```python
from build123d import *

# Parameters (mm, degrees)
SKETCH_1_R      = 2.25
SKETCH_1_R_2    = 2.075
EXTRUDE_1_DEPTH = 2.4
SKETCH_4_R      = 3.5
SKETCH_4_R_2    = 2.075
EXTRUDE_2_DEPTH = 9.9
FILLET_1_R      = 1
SKETCH_5_R      = 2.075
SKETCH_5_R_2    = 1.2
EXTRUDE_3_DEPTH = 4


with BuildPart() as part:
    # 草图1 → 凸台-拉伸1 (new body)
    with BuildSketch(Plane(origin=(0, 0, 0), x_dir=(0, 0, -1), z_dir=(1, 0, 0))):
        with BuildLine():
            Line((-5, 0), (5, 0))
            ThreePointArc((5, 0), (10, 5), (5, 10))
            Line((5, 10), (5, 21.282156306))
            ThreePointArc((5, 21.282156306), (0, 26.282156306), (-5, 21.282156306))
            Line((-5, 21.282156306), (-5, 10))
            ThreePointArc((-5, 10), (-10, 5), (-5, 0))
        make_face()
        with Locations((-5, 5)):
            Circle(SKETCH_1_R, mode=Mode.SUBTRACT)
        with Locations((5, 5)):
            Circle(SKETCH_1_R, mode=Mode.SUBTRACT)
        with Locations((0, 21.282156306)):
            Circle(SKETCH_1_R_2, mode=Mode.SUBTRACT)
    extrude(amount=EXTRUDE_1_DEPTH)

    # 草图4 → 凸台-拉伸2 (add)
    with BuildSketch(Plane(origin=(2.4, 0, 0), x_dir=(0, 0, -1), z_dir=(1, 0, 0))):
        with Locations(Location((0, 21.282156306, 0), (0, 0, 180))):
            Circle(SKETCH_4_R)
        with Locations((0, 21.282156306)):
            Circle(SKETCH_4_R_2, mode=Mode.SUBTRACT)
    extrude(amount=EXTRUDE_2_DEPTH)

    # 圆角1
    fillet_1_edges = [part.edges().sort_by_distance(p)[0] for p in [
        (2.4, 21.282156306, -3.5),
    ]]
    fillet(fillet_1_edges, radius=FILLET_1_R)

    # 草图5 → 凸台-拉伸3 (add)
    with BuildSketch(Plane.ZY):
        with Locations((0, 21.282156306)):
            Circle(SKETCH_5_R)
        with Locations((0, 21.282156306)):
            Circle(SKETCH_5_R_2, mode=Mode.SUBTRACT)
    extrude(amount=-EXTRUDE_3_DEPTH)


solid = part.part
```
For this review, take the finished solid that the model builds, in its own axes (mm). A direction names the side the tool comes from. Coordinates: 2 decimals unless noted, no trailing zeros. Write each loop counter-clockwise with the first axis right and the second up, starting at its lowest first coordinate (ties: lowest second). Pieces come first, ordered by that corner, then holes. Notation, with made-up numbers: (22, 82.5) - (34, 82.5) arc R22 cw to (34, 114.5) - close; hole circle Ø4 at (-27.75, 18.25). An arc over 180 degrees is marked (long way). Put each result on its own line as item: value.
1. For pin 1 (4 mm diameter, centred on y = 21.28, z = 0, fed in from +X); pin 2 (3 mm diameter, centred on x = 6.5, z = -0.5, fed in from -Y); pin 3 (1.2 mm diameter, centred on x = 1.5, y = 18, fed in from -Z); pin 4 (7 mm diameter, centred on y = 5, z = 5, fed in from -X), all flat-tipped, find the tip position at first contact; note any pin that passes through.
Values found:
pin 1: x = 4
pin 2: y = 17.78
pin 3: z = -5
pin 4: x = 0
2. Add section A-A, the plane z = 0. Give the boundary of the cut face in (x, y).
Values found:
outline: (0, 0) - (2.4, 0) - (2.4, 16.78) arc R1 cw to (3.4, 17.78) - (12.3, 17.78) - (12.3, 19.21) - (4, 19.21) - (4, 20.08) - (0, 20.08) - close; (0, 22.48) - (4, 22.48) - (4, 23.36) - (12.3, 23.36) - (12.3, 24.78) - (3.4, 24.78) arc R1 cw to (2.4, 25.78) - (2.4, 26.28) - (0, 26.28) - close
3. Add section B-B, the plane y = 5. Give the boundary of the cut face in (x, z), then the cut area to 3 significant figures.
Values found:
outline: (0, -10) - (2.4, -10) - (2.4, -7.25) - (0, -7.25) - close; (0, -2.75) - (2.4, -2.75) - (2.4, 2.75) - (0, 2.75) - close; (0, 7.25) - (2.4, 7.25) - (2.4, 10) - (0, 10) - close
area: 26.4 mm²
4. Add section D-D, the plane y = 12. Give the boundary of the cut face in (x, z).
Values found:
outline: (0, -5) - (2.4, -5) - (2.4, 5) - (0, 5) - close
5. Machinability: for faces 4 (the flat face through (1, 16, -5)), 5 (the cylindrical face through (1.97, 22.47, -0.16)), 6 (the cylindrical face through (8.092, 19.441, -0.957)), which of the approach directions +Z, -Z, +X, -X, +Y, -Y give a long, thin tool a straight path to every point of the face, cutting with its end or side? Answer none if there is none.
Values found:
face 4: -Z, +X, -X, +Y
face 5: +X, -X
face 6: +X
6. Add section C-C, the plane x = 7.25. Give the boundary of the cut face in (y, z) (3 decimals), then the cut area to 3 significant figures.
Values found:
outline: circle Ø7 at (21.282, 0); hole circle Ø4.15 at (21.282, 0)
area: 25.0 mm²
7. Mouldability with a two-part tool opening along Z and no side actions: class faces 1 (the flat face through (1, 16, 5)), 2 (the flat face through (0, 10, 0)), 3 (the flat face through (4, 20, 1)) as released by +Z, released by -Z, zero draft, split by the parting line, or undercut.
Values found:
face 1: released by +Z
face 2: zero draft
face 3: undercut
8. Wall thickness on probe 1 along Z at (x, y) = (0.5, 5.5); probe 2 along Y at (x, z) = (1.65, 0); probe 3 along Y at (x, z) = (9.5, 0): over which ranges is each line inside the solid? List them lowest first.
Values found:
probe 1: -9.97 to -7.19, -2.81 to 2.81, 7.19 to 9.97
probe 2: 0 to 20.08, 22.48 to 26.28
probe 3: 17.78 to 19.21, 23.36 to 24.78
